Part model, mm, in its own coordinate system. Face numbers are marked on the shaded views. Give positions to 0.01 mm unless a question says otherwise; leave off trailing zeros. Write each loop counter-clockwise with the first axis right and the second up, starting at its lowest first coordinate (ties: lowest second). Pieces come first, ordered by that corner, then holes.
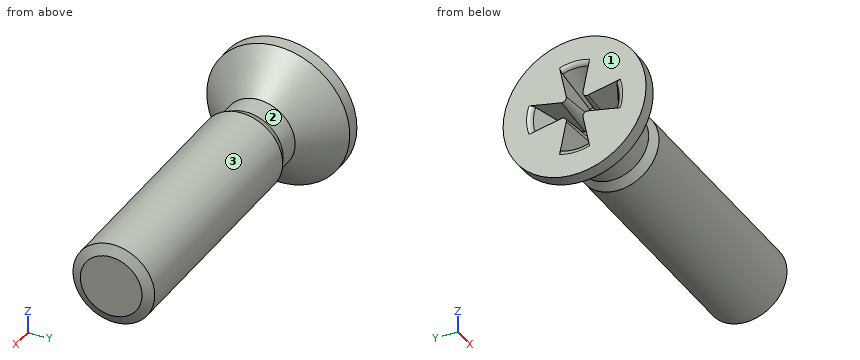
Autodesk Inventor part; units mm, degrees
ref_plane "Work Plane2" through (3.35, 0, 0) normal (0, 0, -1) x (1, 0, 0)
ref_plane "YZ Plane" through (0, 0, 0) normal (1, 0, 0) x (0, 1, 0)
ref_plane "XZ Plane" through (0, 0, 0) normal (0, 1, 0) x (-1, 0, 0)
sketch "Sketch1" plane through (0, 0, 0) normal (0, 0, 1) x (1, 0, 0)
  line L0 (1.32, 0) -> (8, 0)
  line L1 (8, 0) -> (8, 1)
  line L2 (8, 1) -> (2, 1)
  line L3 (2, 1) -> (1.7546, 0.8773)
  line L4 (1.7546, 0.8773) -> (1.2, 0.8773)
  line L5 (0, 1.75) -> (0, 1.09)
  line L6 (0, 1.09) -> (1.0075, 0.5877)
  line L7 (1.0075, 0.5877) -> (1.32, 0)
  line L8 (-1.6, 0) -> (9.6, 0)
  line L9 (0, -0.35) -> (0, 2.1)
  line L10 (0, 1.75) -> (0.3273, 1.75)
  line L11 (0.3273, 1.75) -> (1.2, 0.8773)
  line L12 (2, 1) -> (1.0773, 1) construction
  dimension "d1" = 6
  dimension "d2" = 2
  dimension "d3" = 1.7546
  dimension "d4" = 2.18
  dimension "d5" = 26.5
  dimension "d6" = 62
  dimension "d7" = 1.32
  dimension "d8" = 0.2454
  dimension "d12" = 3.5
  dimension "d13" = 45
  dimension "d15" = 8
  dimension "d24" = 1.2
revolve "Body" add sketch "Sketch1" angle 360 about axis through (1.32, 0, 0) along (1, 0, 0) contours L7 L6 L5 L10 L11 L4 L3 L2 L1 L0
sketch "Sketch2" plane through (0, 0, 0) normal (-1, 0, 0) x (0, 0, 1)
  line L0 (0, 1.09) -> (0, 0) construction
  line L1 (0, 0) -> (1.09, 0) construction
  arc A0 (0.327, 0) -> (0, 0.327) centre (0, 0) ccw construction
  arc A1 (0.3815, 0) -> (0, 0.3815) centre (0, 0) ccw construction
  arc A2 (1.0323, 0.35) -> (0.35, 1.0323) centre (0, 0) ccw
  line L2 (0, 0) -> (0.7707, 0.7707) construction
  line L3 (0.35, 1.0323) -> (0.2039, 0.3225)
  line L4 (1.0323, 0.35) -> (0.3225, 0.2039)
  arc A3 (0.35, 1.0323) -> (0, 1.09) centre (0, 0) ccw
  arc A4 (1.09, 0) -> (1.0323, 0.35) centre (0, 0) ccw
  line L5 (0, -2.45) -> (0, 2.45)
  line L6 (-2.45, 0) -> (2.45, 0)
  arc A5 (0.35, -1.0323) -> (1.0323, -0.35) centre (0, 0) ccw
  line L7 (0.35, -1.0323) -> (0.2039, -0.3225)
  line L8 (1.0323, -0.35) -> (0.3225, -0.2039)
  arc A6 (0, -1.09) -> (0.35, -1.0323) centre (0, 0) ccw
  arc A7 (1.0323, -0.35) -> (1.09, 0) centre (0, 0) ccw
  arc A8 (-0.35, 1.0323) -> (-1.0323, 0.35) centre (0, 0) ccw
  line L9 (-0.35, 1.0323) -> (-0.2039, 0.3225)
  line L10 (-1.0323, 0.35) -> (-0.3225, 0.2039)
  arc A9 (0, 1.09) -> (-0.35, 1.0323) centre (0, 0) ccw
  arc A10 (-1.0323, 0.35) -> (-1.09, 0) centre (0, 0) ccw
  arc A11 (-0.35, -1.0323) -> (0, -1.09) centre (0, 0) ccw
  arc A12 (-1.0323, -0.35) -> (-0.35, -1.0323) centre (0, 0) ccw
  arc A13 (-1.09, 0) -> (-1.0323, -0.35) centre (0, 0) ccw
  line L11 (-1.0323, -0.35) -> (-0.3225, -0.2039)
  line L12 (-0.35, -1.0323) -> (-0.2039, -0.3225)
  arc A14 (0.2039, 0.3225) -> (0.3225, 0.2039) centre (0.3022, 0.3022) ccw
  arc A15 (0.3225, -0.2039) -> (0.2039, -0.3225) centre (0.3022, -0.3022) ccw
  arc A16 (-0.3225, 0.2039) -> (-0.2039, 0.3225) centre (-0.3022, 0.3022) ccw
  arc A17 (-0.2039, -0.3225) -> (-0.3225, -0.2039) centre (-0.3022, -0.3022) ccw
  point P0 (0.7707, -0.7707)
  point P1 (-0.7707, 0.7707)
  point P2 (-0.7707, -0.7707)
  dimension "d17" = 0.654
  dimension "d18" = 0.763
  dimension "d19" = 2.18
  dimension "d20" = 45
  dimension "d21" = 0.35
extrude "Slot" add sketch "Sketch2" against normal up to next draft 5 contours L4 A14 L3 A2 | A5 L7 A15 L8 | L9 A16 L10 A8 | A12 L11 A17 L12
fillet "Fillet1" radius 0.14 4 edges at (0, 1.09, 0) (0, 0, -1.09) (0, -1.09, 0) (0, 0, 1.09)
thread "Thread"
chamfer "Chamfer1" distance 0.2454 distance2 0.1227 1 edges at (8, -1, 0) measured on face at (8, -0.1182, -0.3117)
ref_plane "Work Plane2" through (3.35, 0, 0) normal (0, 0, -1) x (1, 0, 0)
equation "\"d1\" = GEL"
equation "\"d2\" = GD"
equation "\"d3\" = BDM"
equation "\"d4\" = SDM"
equation "\"d7\" = INTI"
equation "\"d8\" = GAL"
equation "\"d12\" = KOD"
equation "\"d13\" = 0.5 * SEWI"
equation "\"d15\" = NLG"
equation "\"d24\" = KOH"
equation "\"d17\" = 0.3 * SDM"
equation "\"d18\" = 0.35 * SDM"
equation "\"d19\" = SDM"
equation "\"d21\" = 0.5 * SBR"
equation "\"d23\" = 0.2 * SBR"
equation "\"d10\" = GEL"
equation "\"d25\" = -0.5 * SPD + 0.5 * GD"
equation "\"d26\" = 0.5 * GAL"
equation "\"NLG\" = 8"
equation "\"GEL\" = 6"
equation "\"GAL\" = 0.61345 * PTC"
equation "\"SPD\" = NND - 1.2269 * PTC"
equation "\"KOD\" = 3.5"
equation "\"KOH\" = 1.2"
equation "\"SBR\" = 0.7"
equation "\"INTI\" = 1.32"
equation "\"SDM\" = 2.18"
equation "\"GD\" = NND"
equation "\"BDM\" = NND - GAL"
equation "\"SEWI\" = 90deg"
equation "\"d9\" = SDM"
equation "\"GUL\" = 0.61345 * PTC"
equation "\"TOA\" = 30deg"
equation "\"EPV\" = 2.2"
equation "\"THREADDIA\" = 2"
equation "\"RR\" = 0.2"
equation "\"PTC\" = 0.4"
equation "\"NND\" = 2"
equation "\"GD1\" = THREADDIA - 1.2269 * PTC"
properties part number "AS 1427 - M2 x 8(5)" material "Steel, Mild"
1) Saw through at A-A (x = 5). Write the cut outline in (y, z), and give its area (3 significant figures).
Check result:
outline: circle Ø2 at (0, 0)
area: 3.14 mm2
2) Drill centre lines: L1, parallel to Z at x = 5.5, y = 0.1; L2, parallel to Z at x = 0.5, y = 0.7; L3, parallel to X at y = -0.6, z = -1.4. Where is each one in solid material? Low to high.
Check result:
L1: z = -0.99 to 0.99
L2: z = -1.41 to -0.24, 0.24 to 1.41
L3: x = 0 to 0.55
3) Mould opens along X. For the marked faces 1, 2 and 3 say: +X half, -X half, draft (parallel to the pull), parting line (faces both ways), or undercut.
Check result:
face 1: -X half
face 2: undercut
face 3: draft
4) Saw through at B-B (x = 1.5). Write the cut outline in (y, z), and give its area (3 significant figures).
Check result:
outline: circle Ø1.75 at (0, 0)
area: 2.42 mm2
5) Flat gauge pins, fed straight in: P1, Ø1, axis at y = 1, z = 1, coming from the +X side; P2, Ø1.5, axis at x = 4, z = 1, coming from the +Y side. Where does each tip first touch, or does it go through?
Check result:
P1: stops at x = 7.92
P2: stops at y = 0.97
